Can you work these out from the drawing? Everything is in mm from the part's minimum corner. Round coordinates to 2 decimals unless told otherwise and drop trailing zeros. Loops run counter-clockwise (first coordinate to the right, second up) from the corner with the lowest first, then second, coordinate; pieces in that order, holes last. Notation, with made-up numbers: (-16, -38.75) -> (22, -38.75) arc R37 cw to (22, -1.75) -> close; hole circle Ø10 at (-12, 48). An arc over 180 degrees is marked (long way). One line per item, written item: value.
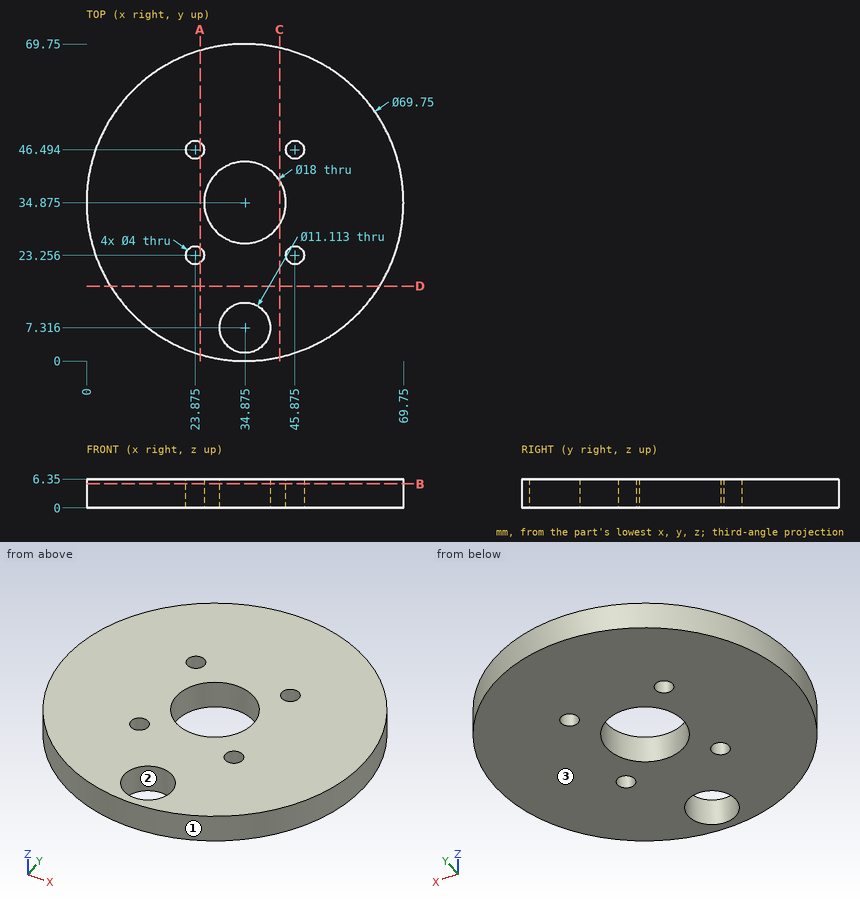
Item 1: If we section it at A-A on x = 25: List the corners of the cut face in (y, z) for me.
Output:
outline: (1.43, 0) -> (21.6, 0) -> (21.6, 6.35) -> (1.43, 6.35) -> close; (24.91, 0) -> (44.84, 0) -> (44.84, 6.35) -> (24.91, 6.35) -> close; (48.15, 0) -> (68.32, 0) -> (68.32, 6.35) -> (48.15, 6.35) -> close
Item 2: If we mould it in two halves opening along Y, with no side actions, what happens to the marked faces 1, 2 and 3? For each: released by +Y, released by -Y, zero draft, split by the parting line, or undercut.
Output:
face 1: split by the parting line
face 2: undercut
face 3: zero draft
Item 3: If we section it at B-B on z = 5.25: Count the separate pieces of the cut face and the enclosed holes in it, plus the area to 3 significant figures.
Output:
separate pieces: 1
enclosed holes: 6
area: 3,420 mm²
Item 4: If we section it at C-C on x = 42.5: List the corners of the cut face in (y, z) for me.
Output:
outline: (0.84, 0) -> (30.09, 0) -> (30.09, 6.35) -> (0.84, 6.35) -> close; (39.66, 0) -> (68.91, 0) -> (68.91, 6.35) -> (39.66, 6.35) -> close
Item 5: I need wall thicknesses on line 1 (Y direction, x = 22.5, z = 3.75) (1 decimal); line 2 (Y direction, x = 47, z = 2.75) (1 decimal); line 3 (X direction, y = 23, z = 0.5) (1 decimal). Which ranges of each line are inside material? Lowest first, please. Write a range as from..to.
Output:
line 1: y = 2.3..21.8, 24.7..45, 47.9..67.5
line 2: y = 2.2..21.6, 24.9..44.8, 48.1..67.6
line 3: x = 2.1..21.9, 25.9..43.9, 47.9..67.7
Item 6: Will these pins go through, and if not, where does the flat tip stop? pin 1 Ø5 at (x, y) = (23.88, 23.26) entering from +Z; pin 2 Ø2 at (x, z) = (62.5, 1.5) entering from +Y; pin 3 Ø1.5 at (y, z) = (37.5, 3) entering from -X; pin 4 Ø3 at (x, y) = (45.88, 46.49) entering from -Z.
Output:
pin 1: stops at z = 6.35
pin 2: stops at y = 57.4
pin 3: stops at x = 0.05
pin 4: passes through
Item 7: If we section it at D-D on y = 16.5: List the corners of the cut face in (x, z) for me.
Output:
outline: (5.23, 0) -> (64.52, 0) -> (64.52, 6.35) -> (5.23, 6.35) -> close
